```python
from build123d import *

# Parameters (mm, degrees)
BOSS_EXTRUDE1_START       = -105
BOSS_EXTRUDE1_DEPTH       = 160
BOSS_EXTRUDE1_2_DEPTH     = 40
BOSS_EXTRUDE1_START_2     = -20
BOSS_EXTRUDE1_3_OUTLINE_W = 47
BOSS_EXTRUDE1_3_OUTLINE_H = 147
BOSS_EXTRUDE1_3_DEPTH     = 20
BOSS_EXTRUDE1_START_3     = 42.132444372
BOSS_EXTRUDE1_4_OUTLINE_W = 53
BOSS_EXTRUDE1_4_OUTLINE_H = 116
BOSS_EXTRUDE1_4_DEPTH     = 19.867555628
BOSS_EXTRUDE1_START_4     = 80.434666527
BOSS_EXTRUDE1_5_OUTLINE_W = 52
BOSS_EXTRUDE1_5_OUTLINE_H = 117
BOSS_EXTRUDE1_5_DEPTH     = 20.565333473
SKETCH3_W                 = 27.900715286
SKETCH3_H                 = 15.750403791
BOSS_EXTRUDE2_DEPTH       = 10
SKETCH4_R                 = 75
CUT_EXTRUDE1_DEPTH        = 80


with BuildPart() as part:
    # Boss-Extrude1: read off the stored shape, not the designer's step
    # Boss-Extrude1 outline → Boss-Extrude1 (new body)
    with BuildSketch(Plane.XY.offset(BOSS_EXTRUDE1_START)):
        Polygon((65, 0), (40, 29.793839815), (15, 0), align=None)
    extrude(amount=BOSS_EXTRUDE1_DEPTH)

    # Boss-Extrude1 2 outline → Boss-Extrude1 2 (add)
    with BuildSketch(Plane.YZ):
        Polygon((0, -50), (29.793839815, -25), (0, 0), align=None)
    extrude(amount=BOSS_EXTRUDE1_2_DEPTH)

    # Boss-Extrude1 3 outline → Boss-Extrude1 3 (cut)
    with BuildSketch(Plane(origin=(0, 0, 0), x_dir=(0.6427876096865404, 0.7660444431189772, 0), z_dir=(0.7660444431189772, -0.6427876096865403, 0)).offset(BOSS_EXTRUDE1_START_2)):
        with Locations((22.5, -24.5)):
            Rectangle(BOSS_EXTRUDE1_3_OUTLINE_W, BOSS_EXTRUDE1_3_OUTLINE_H)
    extrude(amount=BOSS_EXTRUDE1_3_DEPTH, mode=Mode.SUBTRACT)

    # Boss-Extrude1 4 outline → Boss-Extrude1 4 (cut)
    with BuildSketch(Plane(origin=(0, 0, 0), x_dir=(1, 0, 0), z_dir=(0, 0.6427876096865403, 0.7660444431189772)).offset(BOSS_EXTRUDE1_START_3)):
        with Locations((40.5, 21)):
            Rectangle(BOSS_EXTRUDE1_4_OUTLINE_W, BOSS_EXTRUDE1_4_OUTLINE_H)
    extrude(amount=BOSS_EXTRUDE1_4_DEPTH, mode=Mode.SUBTRACT)

    # Boss-Extrude1 5 outline → Boss-Extrude1 5 (cut)
    with BuildSketch(Plane(origin=(0, 0, 0), x_dir=(1, 0, 0), z_dir=(0, 0.6427876096865403, -0.7660444431189772)).offset(BOSS_EXTRUDE1_START_4)):
        with Locations((40, 10.5)):
            Rectangle(BOSS_EXTRUDE1_5_OUTLINE_W, BOSS_EXTRUDE1_5_OUTLINE_H)
    extrude(amount=BOSS_EXTRUDE1_5_DEPTH, mode=Mode.SUBTRACT)

    # Sketch3 → Boss-Extrude2 (add)
    with BuildSketch(Plane.XZ):
        with Locations((-1.039193036, -25.78752019)):
            Rectangle(SKETCH3_W, SKETCH3_H)
    extrude(amount=-BOSS_EXTRUDE2_DEPTH)

    # Sketch4 → Cut-Extrude1 (cut, symmetric)
    with BuildSketch(Plane.XY):
        with Locations((-14.989550679, 85)):
            Circle(SKETCH4_R)
    extrude(amount=CUT_EXTRUDE1_DEPTH, both=True, mode=Mode.SUBTRACT)


solid = part.part
```
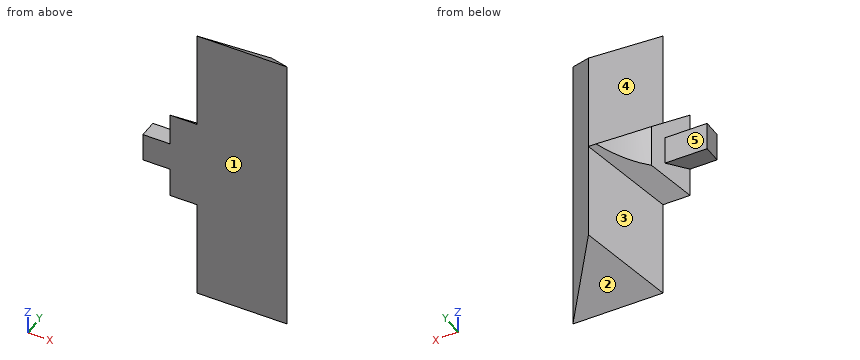
Could you check a few things on this model? Use its own coordinates, in mm. Face numbers are marked on the shaded views. A direction names the side the tool comes from. Round coordinates to 2 decimals unless told otherwise and drop trailing zeros. Order: outer loops, then holes, each group sorted by start corner. A loop starts at its lowest first (then second) coordinate and runs counter-clockwise, first axis right, second up. Notation, with made-up numbers: (-20, 32.5) -> (8, 32.5) arc R35 cw to (8, 69.5) -> close; hole circle Ø10 at (-24, -27). An arc over 180 degrees is marked (long way). One line per question, with ' | ' between items.
Q1. If I drill on line 1 (Y direction, x = 6.5, z = -32); line 2 (Y direction, x = 28.5, z = 1.5); line 3 (Z direction, x = 34.5, y = 19.5), over which ranges is the centre line in solid material (lowest first)? Write a range as from..to.
Computed values:
line 1: 0..10 | line 2: 0..16.09 | line 3: -88.64..38.64
Q2. If we section it at A-A on y = 26.75: Write out the boundary of the cut face in (x, z).
Computed values:
outline: (32.25, -27.55) -> (37.45, -27.55) -> (37.45, -82.55) -> (42.55, -82.55) -> (42.55, 32.55) -> (37.45, 32.55) -> (37.45, -22.45) -> (32.25, -22.45) -> close
Q3. If we section it at C-C on z = -44.5: Write out the boundary of the cut face in (x, y), plus the area to 3 significant figures.
Computed values:
outline: (0, 0) -> (65, 0) -> (40, 29.79) -> (20.5, 6.55) -> (5.5, 6.55) -> close | area: 843 mm²
Q4. If we section it at B-B on x = 20.5: Write out the boundary of the cut face in (y, z), plus the area to 3 significant figures.
Computed values:
outline: (0, -105) -> (6.55, -99.5) -> (6.55, -44.5) -> (18.93, -34.12) -> (18.93, -15.88) -> (6.55, -5.5) -> (6.55, 49.5) -> (0, 55) -> close | area: 1,370 mm²
Q5. If we section it at D-D on y = 3.5: Write out the boundary of the cut face in (x, z), plus the area to 3 significant figures.
Computed values:
outline: (-14.99, -33.66) -> (2.94, -33.66) -> (2.94, -47.06) -> (17.94, -47.06) -> (17.94, -102.06) -> (62.06, -102.06) -> (62.06, 52.06) -> (17.94, 52.06) -> (17.94, -2.94) -> (2.94, -2.94) -> (2.94, -17.91) -> (-14.99, -17.91) -> close | area: 7,750 mm²
Q6. Which directions (+Z, -Z, +X, -X, +Y, -Y) give clear straight access to the entire face, cutting with the end or side of a thin tool? Please do the marked faces 1, 2, 3, 4 and 5.
Computed values:
face 1: +Z, -Z, +X, -X, -Y | face 2: -Z, +X, -X, +Y | face 3: -Z, -X, +Y | face 4: +Z, -X, +Y | face 5: +Z, -Z, -X, +Y
Q7. I'm going to push flat-ended pins straight in: pin 1 (5 mm diameter, centred on x = -5, z = -35.5, fed in from -Y); pin 2 (17.5 mm diameter, centred on x = -8.5, z = -22, fed in from +Y); pin 3 (1 mm diameter, centred on y = 4, z = -35, fed in from +X); pin 4 (3 mm diameter, centred on x = 15, z = -2.5, fed in from +Y). Where does each tip first touch, or does it pass through?
Computed values:
pin 1: y = 0 | pin 2: y = 10 | pin 3: x = 62.06 | pin 4: y = 4.77
